Here's how the part is built. I have some questions about the finished solid (model axes, mm). A direction names the side the tool comes from. Give positions to 0.01 mm unless a question says otherwise; leave off trailing zeros. Loops run counter-clockwise (first coordinate to the right, second up) from the corner with the lowest first, then second, coordinate; pieces in that order, holes last.
Q1. Suppose I cut it at D-D (x = 28.5). List the corners of the cut face in (y, z) for me, and give its area (3 significant figures).
Q2. Suppose I cut it at C-C (y = -5.5). List the corners of the cut face in (x, z) for me, and give its area (3 significant figures).
Q3. Suppose I cut it at B-B (z = 0.75). List the corners of the cut face in (x, y) for me.
Q4. Thinking about a two-plate mould opening in X: for faces 5 (the face through (-0.13, -19.33, 1.48)), 6 (the face through (-32.48, -10.12, 1.48)), 7 (the face through (-16, -20.32, 1)), which applies, pulls with the +X half, pulls with the -X half, needs draft (parallel to the pull), parting line crosses it, or undercut?
Q5. I'm going to push flat-ended pins straight in: P1, Ø0.9, axis at y = 11, z = 1, coming from the +X side; P2, Ø0.9, axis at y = 9, z = 2, coming from the -X side; P3, Ø0.9, axis at x = -26, z = 1.5, coming from the +Y side. Where does each tip first touch, or does it pass through?
Q6. For faces 1 (the face through (-30.48, -16, 1)), 2 (the face through (0, 20.32, 1)), 3 (the face through (26, 20.32, 1)), 4 (the face through (-26, 20.32, 1)), which set-ups out of +Z, -Z, +X, -X, +Y, -Y let a thin tool reach every point of the face, with its end or its side?
Q7. I need wall thicknesses on probe 1 along X at (y, z) = (19, 1.9); probe 2 along Y at (x, z) = (-25.5, 0.75); probe 3 along Y at (x, z) = (-21.5, 1.35). Which ranges of each line are inside material? Lowest first, please.
Q8. Suppose I cut it at A-A (x = 0). List the corners of the cut face in (y, z) for me.
```python
from build123d import *

# Parameters (mm, degrees)
ESQUISSE1_R        = 1
BOSS_EXTRU_2_DEPTH = 3


with BuildPart() as part:
    # Esquisse1 → Boss.-Extru.2 (new body)
    with BuildSketch(Plane.XY):
        with BuildLine():
            Line((30.48, -20.32), (30.48, -12.16))
            ThreePointArc((30.48, -12.16), (32.48, -10.16), (30.48, -8.16))
            Line((30.48, -8.16), (30.48, 20.32))
            Line((30.48, 20.32), (22.32, 20.32))
            ThreePointArc((22.32, 20.32), (20.32, 22.32), (18.32, 20.32))
            Line((18.32, 20.32), (-18.32, 20.32))
            ThreePointArc((-18.32, 20.32), (-20.32, 22.32), (-22.32, 20.32))
            Line((-22.32, 20.32), (-30.48, 20.32))
            Line((-30.48, 20.32), (-30.48, -8.16))
            ThreePointArc((-30.48, -8.16), (-32.48, -10.16), (-30.48, -12.16))
            Line((-30.48, -12.16), (-30.48, -20.32))
            Line((-30.48, -20.32), (-2, -20.32))
            ThreePointArc((-2, -20.32), (0, -22.32), (2, -20.32))
            Line((2, -20.32), (30.48, -20.32))
        make_face()
        with Locations((-30.48, -10.16)):
            Circle(ESQUISSE1_R, mode=Mode.SUBTRACT)
        with Locations((0, -20.32)):
            Circle(ESQUISSE1_R, mode=Mode.SUBTRACT)
        with Locations((30.48, -10.16)):
            Circle(ESQUISSE1_R, mode=Mode.SUBTRACT)
        with Locations((20.32, 20.32)):
            Circle(ESQUISSE1_R, mode=Mode.SUBTRACT)
        with Locations((-20.32, 20.32)):
            Circle(ESQUISSE1_R, mode=Mode.SUBTRACT)
    extrude(amount=BOSS_EXTRU_2_DEPTH)


solid = part.part
```
Solutions:
1. outline: (-20.32, 0) - (20.32, 0) - (20.32, 3) - (-20.32, 3) - close
1. area: 122 mm2
2. outline: (-30.48, 0) - (30.48, 0) - (30.48, 3) - (-30.48, 3) - close
2. area: 183 mm2
3. outline: (-30.48, -20.32) - (-2, -20.32) arc R2 ccw to (2, -20.32) - (30.48, -20.32) - (30.48, -12.16) arc R2 ccw to (30.48, -8.16) - (30.48, 20.32) - (22.32, 20.32) arc R2 ccw to (18.32, 20.32) - (-18.32, 20.32) arc R2 ccw to (-22.32, 20.32) - (-30.48, 20.32) - (-30.48, -8.16) arc R2 ccw to (-30.48, -12.16) - close; hole circle Ø2 at (-30.48, -10.16); hole circle Ø2 at (-20.32, 20.32); hole circle Ø2 at (0, -20.32); hole circle Ø2 at (20.32, 20.32); hole circle Ø2 at (30.48, -10.16)
4. face 5: undercut
4. face 6: pulls with the -X half
4. face 7: needs draft
5. P1: stops at x = 30.48
5. P2: stops at x = -30.48
5. P3: stops at y = 20.32
6. face 1: +Z, -Z, -X, -Y
6. face 2: +Z, -Z, +Y
6. face 3: +Z, -Z, +X, +Y
6. face 4: +Z, -Z, -X, +Y
7. probe 1: x = -30.48 to 30.48
7. probe 2: y = -20.32 to 20.32
7. probe 3: y = -20.32 to 21.93
8. outline: (-22.32, 0) - (-21.32, 0) - (-21.32, 3) - (-22.32, 3) - close; (-19.32, 0) - (20.32, 0) - (20.32, 3) - (-19.32, 3) - close
